from build123d import *

# Parameters (mm, degrees)
BOSS_EXTRUDE1_DEPTH     = 65
CUT_EXTRUDE1_DEPTH      = 188.52539512587924
CUT_EXTRUDE1_DEPTH_BACK = 188.52539512587924
CUT_EXTRUDE2_DEPTH      = 188.52539512587933
CUT_EXTRUDE2_DEPTH_BACK = 188.52539512587933
SHELL2_T                = -1.5
BOSS_EXTRUDE2_DEPTH     = 20
SKETCH8_R               = 7.5
CUT_EXTRUDE3_DEPTH      = 20
BOSS_EXTRUDE4_DEPTH     = 5
FILLET12_R              = 10


with BuildPart() as part:
    # Sketch1 → Boss-Extrude1 (new body)
    with BuildSketch(Plane(origin=(0, 0, 0), x_dir=(0, 0, -1), z_dir=(1, 0, 0))):
        with BuildLine():
            Line((-106.35767816643843, 0), (163.6423218335616, 0))
            Line((163.6423218335616, 0), (173.6423218335616, 9.7979589711327))
            Line((173.6423218335616, 9.7979589711327), (-66.35767816643839, 28.050095))
            ThreePointArc((-66.35767816643839, 28.050095), (-91.13754828258394, 20.841238484230953), (-106.35767816643843, 0))
        make_face()
    extrude(amount=BOSS_EXTRUDE1_DEPTH)

    # Sketch3 → Cut-Extrude1 (cut, two sides: drawn at the far end of the back side and taken through both)
    with BuildSketch(Plane.XZ.offset(-CUT_EXTRUDE1_DEPTH_BACK)):
        Polygon((-72.93745664211396, 555.916712807033), (0, -16.642321833561624), (19.999999999999996, -173.6423218335616), (92.93745664211396, -746.2013564741562), (-1052.1806126390752, -892.0762697583841), (-1218.0555259233033, 410.04179952280515), align=None)
    extrude(amount=CUT_EXTRUDE1_DEPTH + CUT_EXTRUDE1_DEPTH_BACK, mode=Mode.SUBTRACT)

    # Sketch5 → Cut-Extrude2 (cut, two sides: drawn at the far end of the back side and taken through both)
    with BuildSketch(Plane.XZ.offset(-CUT_EXTRUDE2_DEPTH_BACK)):
        Polygon((137.93745664211394, 555.916712807033), (65, -16.64232183356158), (45, -173.6423218335616), (-27.937456642113958, -746.2013564741562), (1117.1806126390752, -892.0762697583841), (1283.0555259233033, 410.04179952280515), align=None)
    extrude(amount=CUT_EXTRUDE2_DEPTH + CUT_EXTRUDE2_DEPTH_BACK, mode=Mode.SUBTRACT)

    # Shell2
    shell2_openings = [part.faces().sort_by_distance(p)[0] for p in [
        (32.5, 20.220874291, -36.589887377),
        (32.5, 20.841238484, 91.137548283),
    ]]
    offset(amount=SHELL2_T, openings=shell2_openings, kind=Kind.INTERSECTION)

    # Sketch7 → Boss-Extrude2 (add)
    with BuildSketch(Plane(origin=(0, 1.5, 0), x_dir=(1, 0, 0), z_dir=(0, 1, 0))):
        Polygon((22.499999999999993, -71.3649853274635), (42.49999999999999, -71.3649853274635), (42.5, -89.36498532746351), (22.499999999999996, -89.36498532746351), align=None)
    extrude(amount=BOSS_EXTRUDE2_DEPTH)

    # Sketch8 → Cut-Extrude3 (cut)
    with BuildSketch(Plane.XY.offset(89.36498532746351)):
        with Locations((32.49999999999999, 11.500000000000002)):
            Circle(SKETCH8_R)
    extrude(amount=-CUT_EXTRUDE3_DEPTH, mode=Mode.SUBTRACT)

    # Sketch18 → Boss-Extrude4 (add)
    with BuildSketch(Plane.XZ):
        Polygon((65, 106.35767816643843), (0, 106.35767816643843), (0, -16.642321833561624), (18.726114649681534, -163.6423218335616), (46.27388535031847, -163.6423218335616), (65, -16.64232183356158), align=None)
    extrude(amount=BOSS_EXTRUDE4_DEPTH)

    # Fillet12
    fillet12_edges = [part.edges().sort_by_distance(p)[0] for p in [
        (65, -5, 44.857678166438426),
        (0, -5, 44.857678166438404),
        (9.363057324840767, -5, -90.14232183356161),
        (55.63694267515924, -5, -90.1423218335616),
    ]]
    fillet(fillet12_edges, radius=FILLET12_R)


solid = part.part
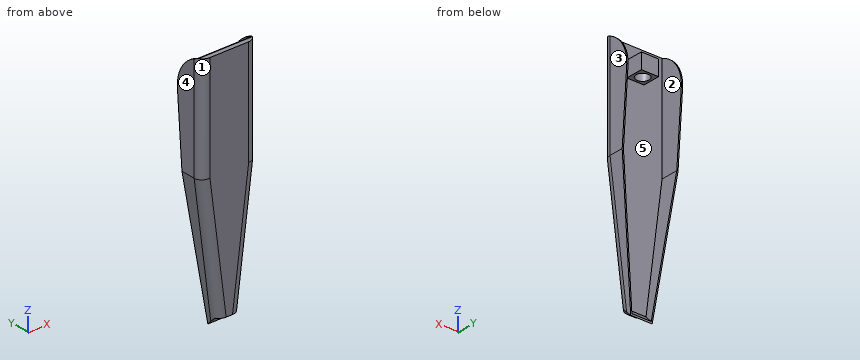
Read the model definition and answer for the solid it produces. Units are mm, in the model's axes. Face numbers are marked on the shaded views. A direction names the side the tool comes from. Coordinates: 2 decimals unless noted, no trailing zeros. Order: outer loops, then holes, each group sorted by start corner. A loop starts at its lowest first (then second) coordinate and runs counter-clockwise, first axis right, second up. Notation, with made-up numbers: (-2.75, 53.5) -> (49.25, 53.5) arc R26 cw to (49.25, 80.5) -> close; hole circle Ø5 at (-28.5, 29). An arc over 180 degrees is marked (long way). Answer as a JSON object with one key per item and string values.
1) Consider line 1 along X through (y, z) = (11, 84); line 2 along Y through (x, z) = (32, 85); line 3 along X through (y, z) = (25, 56.5). Determine where each line is inside the solid, lowest interval first. Write a range as from..to.
Model answer:
{"line 1": "x = 0..1.5, 22.5..25.02, 39.98..42.5, 63.5..65", "line 2": "y = -5..4.02, 18.98..21.5", "line 3": "x = 0..1.5, 63.5..65"}
2) Each of these flat-tipped pins is pushed along its axis until it touches: pin 1 (3 mm diameter, centred on y = 3, z = -9.5, fed in from -X); pin 2 (10 mm diameter, centred on x = 36.5, y = 11, fed in from +Z) (3 decimals); pin 3 (4 mm diameter, centred on y = -1.5, z = -31, fed in from -X). Where does it stop, or does it pass through?
Model answer:
{"pin 1": "stops at x = 0.01", "pin 2": "stops at z = 89.365", "pin 3": "stops at x = 2.88"}
3) A cutting plane is placed at B-B, the plane z = 23.5. Determine the outline of the cut face in (x, y), plus the area to 3 significant figures.
Model answer:
{"outline": "(0, 5) arc R10 ccw to (10, -5) -> (55, -5) arc R10 ccw to (65, 5) -> (65, 24.79) -> (63.5, 24.79) -> (63.5, 1.5) -> (1.5, 1.5) -> (1.5, 24.79) -> (0, 24.79) -> close", "area": "449 mm²"}
4) A tool of negligible diameter and unlimited length cuts with its end or side. For the marked faces 1 and 2, from which of +Z, -Z, +X, -X, +Y, -Y can it reach the whole face along a straight path? Write none if from no direction.
Model answer:
{"face 1": "+Z, -Z, -X, -Y", "face 2": "+Z, +Y"}
5) A cutting plane is placed at A-A, the plane x = 32.5. Determine the outline of the cut face in (y, z), plus the area to 3 significant figures.
Model answer:
{"outline": "(-5, -163.64) -> (0, -163.64) -> (9.8, -173.64) -> (9.95, -171.65) -> (1.5, -163.03) -> (1.5, 71.36) -> (4, 71.36) -> (4, 89.36) -> (1.5, 89.36) -> (1.5, 105.86) arc R40 ccw to (0, 106.36) -> (-5, 106.36) -> close; (19, 71.36) -> (21.5, 71.36) -> (21.5, 89.36) -> (19, 89.36) -> close", "area": "1,860 mm²"}
6) The mould has two halves that part along X. Classify the marked faces 3, 4 and 5: released by +X, released by -X, zero draft, split by the parting line, or undercut.
Model answer:
{"face 3": "released by +X", "face 4": "released by -X", "face 5": "undercut"}
